from build123d import *

# Parameters (mm, degrees)
F0_R     = 12
F1_DEPTH = 2
F3_DEPTH = 25


with BuildPart() as f1:
    # F0 (on Top) → F1 (new body)
    with BuildSketch(Plane.XY):
        Circle(F0_R)
    extrude(amount=F1_DEPTH)

    # F2 (on face) → F3 (cut)
    with BuildSketch(Plane.XY.offset(2)):
        with BuildLine():
            Line((-6.5106279217, -1.8662924413), (-6.5106279217, 2.4396951776))
            Line((-6.5106279217, 2.4396951776), (-6.4994953498, 2.4396951776))
            Line((-6.4994953498, 2.4396951776), (-6.4994953498, 4.2018918664))
            Line((-6.4994953498, 4.2018918664), (-5.0467973821, 4.2018918664))
            add(Edge.make_bspline(
                [(-3.2430132195, 3.7814293576), (-3.8043306687, 4.2018918664), (-5.0467973821, 4.2018918664)],
                knots=[0, 0, 0, 1, 1, 1], degree=2))
            add(Edge.make_bspline(
                [(-2.6816957703, 2.4086192665), (-2.6816957703, 3.3609668488), (-3.2430132195, 3.7814293576)],
                knots=[0, 0, 0, 1, 1, 1], degree=2))
            add(Edge.make_bspline(
                [(-3.233552813, 0.9990187059), (-2.6816957703, 1.4688855594), (-2.6816957703, 2.4086192665)],
                knots=[0, 0, 0, 1, 1, 1], degree=2))
            add(Edge.make_bspline(
                [(-4.5059826225, 0.5491711407), (-3.6714994229, 0.6261384495), (-3.233552813, 0.9990187059)],
                knots=[0.2064129368, 0.2064129368, 0.2064129368, 1, 1, 1], degree=2))
            Line((-4.5059826225, 0.5491711407), (-4.5059826225, -0.4295026676))
            Line((-4.5059826225, -0.4295026676), (-4.493889183, -0.4295026676))
            Line((-4.493889183, -0.4295026676), (-2.1687315096, -4.4238965008))
            Line((-2.1687315096, -4.4238965008), (-0.8484792321, -4.4238965008))
            Line((-0.8484792321, -4.4238965008), (-3.4574490989, -0.1078488484))
            add(Edge.make_bspline(
                [(-1.5254238712, 2.4674840177), (-1.5254238712, 0.562788853), (-3.4574490989, -0.1078488484)],
                knots=[0, 0, 0, 1, 1, 1], degree=2))
            add(Edge.make_bspline(
                [(-2.3695023575, 4.5046248727), (-1.5254238712, 3.8276802336), (-1.5254238712, 2.4674840177)],
                knots=[0, 0, 0, 1, 1, 1], degree=2))
            add(Edge.make_bspline(
                [(-4.9816256932, 5.1815695118), (-3.2135808439, 5.1815695118), (-2.3695023575, 4.5046248727)],
                knots=[0, 0, 0, 1, 1, 1], degree=2))
            Line((-4.9816256932, 5.1815695118), (-7.6158233106, 5.1815695118))
            Line((-7.6158233106, 5.1815695118), (-7.6158233106, -4.4238965008))
            Line((-7.6158233106, -4.4238965008), (-6.4994953498, -4.4238965008))
            Line((-6.4994953498, -4.4238965008), (-6.4994953498, -1.8662924413))
            Line((-6.4994953498, -1.8662924413), (-6.5106279217, -1.8662924413))
        make_face()
        with BuildLine():
            Line((8.1914647062, 0.609039729), (4.9265733257, 0.609039729))
            Line((4.9265733257, 0.609039729), (4.9265733257, -0.3895587293))
            Line((4.9265733257, -0.3895587293), (7.0730344329, -0.3895587293))
            Line((7.0730344329, -0.3895587293), (7.0730344329, -3.3454101659))
            add(Edge.make_bspline(
                [(5.1220883923, -3.5766645457), (6.1206868506, -3.5766645457), (7.0730344329, -3.3454101659)],
                knots=[0, 0, 0, 1, 1, 1], degree=2))
            add(Edge.make_bspline(
                [(2.3333708029, -2.5717591498), (3.2825649165, -3.5766645457), (5.1220883923, -3.5766645457)],
                knots=[0, 0, 0, 1, 1, 1], degree=2))
            add(Edge.make_bspline(
                [(1.3841766894, 0.3777853492), (1.3841766894, -1.5668537538), (2.3333708029, -2.5717591498)],
                knots=[0, 0, 0, 1, 1, 1], degree=2))
            add(Edge.make_bspline(
                [(2.3701612725, 3.2758231908), (1.3841766894, 2.2320250128), (1.3841766894, 0.3777853492)],
                knots=[0, 0, 0, 1, 1, 1], degree=2))
            add(Edge.make_bspline(
                [(5.109474517, 4.3196213688), (3.3561458555, 4.3196213688), (2.3701612725, 3.2758231908)],
                knots=[0, 0, 0, 1, 1, 1], degree=2))
            add(Edge.make_bspline(
                [(7.6133287567, 3.7688154823), (6.3119972921, 4.3196213688), (5.109474517, 4.3196213688)],
                knots=[0, 0, 0, 1, 1, 1], degree=2))
            Line((7.6133287567, 3.7688154823), (8.0464051407, 4.7548000654))
            add(Edge.make_bspline(
                [(5.1809531435, 5.3182198271), (6.7198459256, 5.3182198271), (8.0464051407, 4.7548000654)],
                knots=[0, 0, 0, 1, 1, 1], degree=2))
            add(Edge.make_bspline(
                [(2.5351928071, 4.7243165335), (3.6651857994, 5.3182198271), (5.1809531435, 5.3182198271)],
                knots=[0, 0, 0, 1, 1, 1], degree=2))
            add(Edge.make_bspline(
                [(0.8039384273, 3.0035737164), (1.4051998149, 4.1304132399), (2.5351928071, 4.7243165335)],
                knots=[0, 0, 0, 1, 1, 1], degree=2))
            add(Edge.make_bspline(
                [(0.2026770398, 0.3777853492), (0.2026770398, 1.8767341929), (0.8039384273, 3.0035737164)],
                knots=[0, 0, 0, 1, 1, 1], degree=2))
            add(Edge.make_bspline(
                [(1.4178136901, -3.2581641953), (0.2026770398, -1.9599861995), (0.2026770398, 0.3777853492)],
                knots=[0, 0, 0, 1, 1, 1], degree=2))
            add(Edge.make_bspline(
                [(4.8130484484, -4.5563421911), (2.6329503404, -4.5563421911), (1.4178136901, -3.2581641953)],
                knots=[0, 0, 0, 1, 1, 1], degree=2))
            add(Edge.make_bspline(
                [(6.6399580489, -4.4312545947), (5.851590845, -4.5563421911), (4.8130484484, -4.5563421911)],
                knots=[0, 0, 0, 1, 1, 1], degree=2))
            add(Edge.make_bspline(
                [(8.1914647062, -4.0622987433), (7.4283252528, -4.3061669984), (6.6399580489, -4.4312545947)],
                knots=[0, 0, 0, 1, 1, 1], degree=2))
            Line((8.1914647062, -4.0622987433), (8.1914647062, 0.609039729))
        make_face()
    extrude(amount=-F3_DEPTH, mode=Mode.SUBTRACT)


solid = f1.part
Geometry check sheet. Reference: the model listing, model coordinates, mm. Round coordinates to 2 decimals unless told otherwise and drop trailing zeros. Loops run counter-clockwise (first coordinate to the right, second up) from the corner with the lowest first, then second, coordinate; pieces in that order, holes last. Notation, with made-up numbers: (50, 3) -> (96, 3) arc R20 cw to (96, 10) -> close; hole circle Ø11 at (19.25, 17.5). An arc over 180 degrees is marked (long way). Answer as a JSON object with one key per item and string values. Group by question number.
Item 1: Cross-section at B-B, the plane y = 10.25. Record the cut outline in (x, z), plus the area to 3 significant figures.
Item 2: Thickness scan on line 1 along Y through (x, z) = (7.75, 0.2); line 2 along Y through (x, z) = (2.75, 0.3); line 3 along Y through (x, z) = (-3.25, 1.6). Record the ranges inside material, lowest first.
Item 3: Depth check by flat-ended pin: pin 1 Ø0.6 at (y, z) = (0.5, 0.5) entering from -X; pin 2 Ø3 at (x, y) = (7, 7) entering from -Z; pin 3 Ø1 at (x, z) = (-3, 0.5) entering from +Y; pin 4 Ø1 at (x, z) = (-6.5, 1) entering from -Y. Enter the tip coordinate at first touch or a pass-through.
Item 4: Release check for a two-part mould opening along Y. For faces 1 (the face through (-11.99, 0.53, 0.99)), 2 (the face through (0, 0, 2)), 3 (the face through (7.073, -2, 1)) record: pulls with the +Y half, pulls with the -Y half, needs draft (parallel to the pull), parting line crosses it, or undercut.
Item 5: Cross-section at C-C, the plane x = -8.75. Record the cut outline in (y, z).
Item 6: Cross-section at A-A, the plane z = 1.3. Count the separate pieces of the cut face and the enclosed holes in it, plus the area to 3 significant figures.
Determined:
{
 "1": {"outline": "(-6.24, 0) -> (6.24, 0) -> (6.24, 2) -> (-6.24, 2) -> close", "area": "25.0 mm²"},
 "2": {"line 1": "y = -9.16 to -4.19, 0.61 to 4.08, 4.87 to 9.16", "line 2": "y = -11.68 to -4.18, -2.93 to 3.62, 4.83 to 11.68", "line 3": "y = -11.55 to -2.57, -0.45 to -0.03, 0.99 to 3.79, 4.96 to 11.55"},
 "3": {"pin 1": "stops at x = -12", "pin 2": "stops at z = 0", "pin 3": "stops at y = 11.74", "pin 4": "stops at y = -10.39"},
 "4": {"face 1": "parting line crosses it", "face 2": "needs draft", "face 3": "undercut"},
 "5": {"outline": "(-8.21, 0) -> (8.21, 0) -> (8.21, 2) -> (-8.21, 2) -> close"},
 "6": {"separate pieces": "1", "enclosed holes": "2", "area": "399 mm²"}
}
